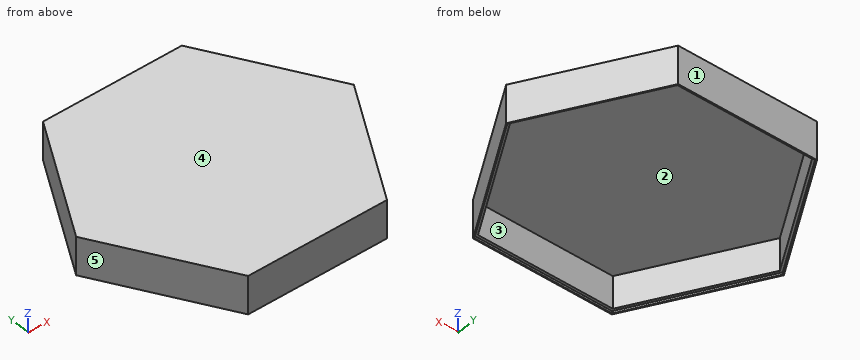
```python
from build123d import *

# Parameters (mm, degrees)
BOSS_EXTRU_1_DEPTH      = 1.5
ESQUISSE3_W             = 15
ESQUISSE3_H             = 60
BOSS_EXTRU_2_DEPTH      = 1.5
ESQUISSE5_W             = 60
ESQUISSE5_H             = 15
BOSS_EXTRU_3_DEPTH      = 1.5
ESQUISSE6_W             = 15
ESQUISSE6_H             = 60
BOSS_EXTRU_4_DEPTH      = 1.5
ENL_V_MAT_EXTRU_1_DEPTH = 1


with BuildPart() as part:
    # Esquisse1 → Boss.-Extru.1 (new body)
    with BuildSketch(Plane.XY):
        Polygon((-30, -51.961524227), (30, -51.961524227), (60, 0), (30, 51.961524227), (-30, 51.961524227), (-60, 0), align=None)
    extrude(amount=BOSS_EXTRU_1_DEPTH)

    # Esquisse3 → Boss.-Extru.2 (add)
    with BuildSketch(Plane(origin=(-45, -25.980762114, 0), x_dir=(0, 0, 1), z_dir=(-0.8660254037844386, -0.5000000000000001, 0))):
        with Locations((-7.5, 0)):
            Rectangle(ESQUISSE3_W, ESQUISSE3_H)
    boss_extru_2 = extrude(amount=-BOSS_EXTRU_2_DEPTH)

    # Esquisse5 → Boss.-Extru.3 (add)
    with BuildSketch(Plane(origin=(0, -51.961524227, 0), x_dir=(-1, 0, 0), z_dir=(0, -1, 0))):
        with Locations((0, 7.5)):
            Rectangle(ESQUISSE5_W, ESQUISSE5_H)
    boss_extru_3 = extrude(amount=-BOSS_EXTRU_3_DEPTH)

    # Esquisse6 → Boss.-Extru.4 (add)
    with BuildSketch(Plane(origin=(45, -25.980762114, 0), x_dir=(0, 0, -1), z_dir=(0.8660254037844389, -0.4999999999999996, 0))):
        with Locations((7.5, 0)):
            Rectangle(ESQUISSE6_W, ESQUISSE6_H)
    boss_extru_4 = extrude(amount=-BOSS_EXTRU_4_DEPTH)

    # Symétrie1: Boss.-Extru.2, Boss.-Extru.3, Boss.-Extru.4 across plane
    add(boss_extru_2.mirror(Plane.ZX))
    add(boss_extru_3.mirror(Plane.ZX))
    add(boss_extru_4.mirror(Plane.ZX))

    # Esquisse7 → Enlèv. mat.-Extru.1 (cut)
    with BuildSketch(Plane(origin=(0, 0, -15), x_dir=(-1, 0, 0), z_dir=(0, 0, -1))):
        Polygon((-59.5, 0), (-29.75, -51.528511525), (29.75, -51.528511525), (59.5, 0), (29.75, 51.528511525), (-29.75, 51.528511525), align=None)
    extrude(amount=-ENL_V_MAT_EXTRU_1_DEPTH, mode=Mode.SUBTRACT)


solid = part.part
```
Check sheet for the modelled part. Datum: model origin and axes. Units: mm. Face numbers are marked on the shaded views. A direction names the side the tool comes from. Give positions to 0.01 mm unless a question says otherwise; leave off trailing zeros. Order: outer loops, then holes, each group sorted by start corner. A loop starts at its lowest first (then second) coordinate and runs counter-clockwise, first axis right, second up. Notation, with made-up numbers: (46, 12.25) -> (73, 12.25) arc R22 ccw to (73, 32.25) -> close; hole circle Ø1 at (-24.5, 87.5). An arc over 180 degrees is marked (long way). Use CSV: the item, a comma, the result in double quotes. Start each with the question number.
1) Set-up check for the marked faces 1 and 2: record each of +Z, -Z, +X, -X, +Y, -Y from which the full face is reachable in a straight line by a thin tool's end or side.
2) Sectioned sample at A-A, the plane z = -1.5. Record the boundary of the cut face in (x, y), plus the area to 3 significant figures.
3) Mould release check, pull along Y, two halves, no side actions. Record for the marked faces 3, 4 and 5: released by +Y, released by -Y, zero draft, split by the parting line, or undercut.
4) Sectioned sample at B-B, the plane x = -9. Record the boundary of the cut face in (y, z), plus the area to 3 significant figures.
5) Go/stop test with flat-tipped pins: P1, Ø4, axis at y = 0.5, z = -6, coming from the -X side; P2, Ø1.5, axis at y = 21.5, z = -6, coming from the +X side; P3, Ø6, axis at x = 45.5, z = -9, coming from the -Y side. Record where each tip stops, or that it passes through.
6) Sectioned sample at C-C, the plane y = 6. Record the boundary of the cut face in (x, z), plus the area to 3 significant figures.
7) Material ranges on line 1 (Y direction, x = 22, z = -2); line 2 (Z direction, x = -45, y = -20); line 3 (X direction, y = 15.5, z = -12.75), recorded low to high. Write a range as from..to.
Recorded:
1,face 1,"+Z, -Z, +X, -X, +Y"
1,face 2,"-Z"
2,outline,"(-60, 0) -> (-30, -51.96) -> (30, -51.96) -> (60, 0) -> (30, 51.96) -> (-30, 51.96) -> close; hole (-58.27, 0) -> (-29.13, -50.46) -> (29.13, -50.46) -> (58.27, 0) -> (29.13, 50.46) -> (-29.13, 50.46) -> close"
2,area,"532 mm2"
3,face 3,"undercut"
3,face 4,"zero draft"
3,face 5,"released by -Y"
4,outline,"(-51.96, -15) -> (-51.53, -15) -> (-51.53, -14) -> (-50.46, -14) -> (-50.46, 0) -> (50.46, 0) -> (50.46, -14) -> (51.53, -14) -> (51.53, -15) -> (51.96, -15) -> (51.96, 1.5) -> (-51.96, 1.5) -> close"
4,area,"199 mm2"
5,P1,"x = -60"
5,P2,"x = 48.02"
5,P3,"y = -30.31"
6,outline,"(-56.54, -15) -> (-56.04, -15) -> (-56.04, -14) -> (-54.8, -14) -> (-54.8, 0) -> (54.8, 0) -> (54.8, -14) -> (56.04, -14) -> (56.04, -15) -> (56.54, -15) -> (56.54, 1.5) -> (-56.54, 1.5) -> close"
6,area,"219 mm2"
7,line 1,"-51.96..-50.46, 50.46..51.96"
7,line 2,"0..1.5"
7,line 3,"-51.05..-49.32, 49.32..51.05"
